Autodesk Inventor part; units mm, degrees
ref_plane "YZ Plane" through (0, 0, 0) normal (1, 0, 0) x (0, 1, 0)
ref_plane "XZ Plane" through (0, 0, 0) normal (0, 1, 0) x (-1, 0, 0)
ref_plane "XY Plane" through (0, 0, 0) normal (0, 0, 1) x (1, 0, 0)
ref_plane "Work Plane1" through (228.6, 0, -127) normal (0, 0, -1) x (-1, 0, 0)
sketch "Sketch5" plane through (228.6, 0, -127) normal (0, 0, -1) x (-1, 0, 0)
  line L0 (0, 0) -> (228.6, 0)
  line L1 (228.6, 0) -> (228.6, 194.818)
  line L2 (228.6, 194.818) -> (0, 194.818)
  line L3 (0, 194.818) -> (0, 0)
  circle A0 centre (549.0601, -0.0332) radius 2.1647 construction
  circle A1 centre (192.2498, 69.0594) radius 2.1647 construction
  arc A2 (37.5756, 109.1194) -> (31.2075, 73.1741) centre (549.0601, -0.0332) ccw construction
  arc A3 (33.8495, 109.9145) -> (27.435, 73.7074) centre (549.0601, -0.0332) ccw
  arc A4 (41.3017, 108.3242) -> (34.98, 72.6408) centre (549.0601, -0.0332) ccw
  arc A5 (41.3017, 108.3242) -> (33.8495, 109.9145) centre (37.5756, 109.1194) ccw
  arc A6 (27.435, 73.7074) -> (34.98, 72.6408) centre (31.2075, 73.1741) ccw
  line L4 (549.0601, -0.0332) -> (37.5756, 109.1194) construction
  line L5 (549.0601, -0.0332) -> (31.2075, 73.1741) construction
  arc A7 (14.9709, 119.3205) -> (7.984, 69.4017) centre (192.2498, 69.0594) ccw construction
  arc A8 (11.3053, 120.3597) -> (4.174, 69.4087) centre (192.2498, 69.0594) ccw
  arc A9 (18.6364, 118.2812) -> (11.794, 69.3946) centre (192.2498, 69.0594) ccw
  arc A10 (18.6364, 118.2812) -> (11.3053, 120.3597) centre (14.9709, 119.3205) ccw
  arc A11 (4.174, 69.4087) -> (11.794, 69.3946) centre (7.984, 69.4017) ccw
  circle A12 centre (192.2498, 69.0594) radius 2.1647
  circle A13 centre (216.5947, 65.3523) radius 2.2284
  line L6 (0, 0) -> (25.4, 0) construction
  line L7 (25.4, 0) -> (25.4, 25.4) construction
  line L8 (25.4, 25.4) -> (0, 25.4) construction
  line L9 (0, 25.4) -> (0, 0) construction
  line L10 (228.6, 0) -> (203.2, 0) construction
  line L11 (203.2, 0) -> (203.2, 25.4) construction
  line L12 (203.2, 25.4) -> (228.6, 25.4) construction
  line L13 (228.6, 25.4) -> (228.6, 0) construction
  line L14 (25.4, 25.4) -> (0, 0) construction
  line L15 (0, 25.4) -> (25.4, 0) construction
  line L16 (203.2, 25.4) -> (228.6, 0) construction
  line L17 (228.6, 25.4) -> (203.2, 0) construction
  circle A14 centre (12.7, 12.7) radius 2.3813
  circle A15 centre (215.9, 12.7) radius 2.3812
  line L18 (228.6, 194.818) -> (222.25, 194.818) construction
  line L19 (222.25, 194.818) -> (222.25, 169.418) construction
  line L20 (222.25, 169.418) -> (228.6, 169.418) construction
  line L21 (228.6, 169.418) -> (228.6, 194.818) construction
  line L22 (222.25, 194.818) -> (196.85, 194.818) construction
  line L23 (222.25, 169.418) -> (222.25, 194.818) construction
  line L24 (196.85, 194.818) -> (107.95, 194.818) construction
  line L25 (107.95, 194.818) -> (133.35, 194.818) construction
  line L26 (222.25, 194.818) -> (209.55, 194.818) construction
  line L27 (209.55, 194.818) -> (209.55, 182.118) construction
  line L28 (209.55, 182.118) -> (222.25, 182.118) construction
  line L29 (222.25, 182.118) -> (222.25, 194.818) construction
  line L30 (209.55, 194.818) -> (146.05, 194.818) construction
  line L31 (146.05, 194.818) -> (158.75, 194.818) construction
  line L32 (158.75, 194.818) -> (158.75, 182.118) construction
  line L33 (158.75, 182.118) -> (146.05, 182.118) construction
  line L34 (146.05, 182.118) -> (146.05, 194.818) construction
  line L35 (222.25, 194.818) -> (209.55, 182.118) construction
  line L36 (209.55, 194.818) -> (222.25, 182.118) construction
  line L37 (158.75, 194.818) -> (146.05, 182.118) construction
  line L38 (158.75, 182.118) -> (146.05, 194.818) construction
  circle A16 centre (215.9, 188.468) radius 2.3812
  circle A17 centre (152.4, 188.468) radius 2.3812
  dimension "d16" = 228.6
  dimension "d17" = 194.818
  dimension "d38" = 4
  dimension "d39" = 7.62
  dimension "d40" = 7.62
  dimension "d43" = 25.4
  dimension "d44" = 25.4
  dimension "d45" = 25.4
  dimension "d46" = 25.4
  dimension "d47" = 4.7625
  dimension "d48" = 4.7625
  dimension "d61" = 6.35
  dimension "d70" = 12.7
  dimension "d71" = 12.7
  dimension "d72" = 63.5
  dimension "d73" = 12.7
  dimension "d74" = 12.7
  dimension "d75" = 4.7625
  dimension "d76" = 4.7625
extrude "Extrusion5" add sketch "Sketch5" along normal blind 3.175
ref_plane "Work Plane2" through (0, 0.0003, -127) normal (-1, 0, 0) x (0, 0, 1)
sketch "Sketch6" plane through (0, 0.0003, -127) normal (-1, 0, 0) x (0, 0, 1)
  line L0 (-3.175, -0.0003) -> (-3.175, 194.8177)
  line L1 (-3.175, 194.8177) -> (127, 194.8177)
  line L2 (127, 194.8177) -> (127, -0.0003)
  line L3 (127, -0.0003) -> (-3.175, -0.0003)
  line L4 (-3.175, -0.0003) -> (-3.175, 194.8177)
  line L5 (0, -0.0003) -> (0, 194.8177) construction
  line L6 (0, -0.0003) -> (25.4, -0.0003) construction
  line L7 (25.4, -0.0003) -> (25.4, 25.3997) construction
  line L8 (25.4, 25.3997) -> (0, 25.3997) construction
  line L9 (0, 25.3997) -> (0, -0.0003) construction
  line L10 (127, -0.0003) -> (101.6, -0.0003) construction
  line L11 (101.6, -0.0003) -> (101.6, 25.3997) construction
  line L12 (101.6, 25.3997) -> (127, 25.3997) construction
  line L13 (127, 25.3997) -> (127, -0.0003) construction
  line L14 (0, -0.0003) -> (25.4, 25.3997) construction
  line L15 (0, 25.3997) -> (25.4, -0.0003) construction
  line L16 (101.6, -0.0003) -> (127, 25.3997) construction
  line L17 (101.6, 25.3997) -> (127, -0.0003) construction
  circle A0 centre (12.7, 12.6997) radius 2.3813
  circle A1 centre (114.3, 12.6997) radius 2.3813
  line L18 (0, 194.8177) -> (3.175, 194.8177) construction
  line L19 (3.175, 194.8177) -> (3.175, 169.4177) construction
  line L20 (3.175, 169.4177) -> (0, 169.4177) construction
  line L21 (0, 169.4177) -> (0, 194.8177) construction
  line L22 (3.175, 194.8177) -> (15.875, 194.8177) construction
  line L23 (15.875, 194.8177) -> (15.875, 182.1177) construction
  line L24 (15.875, 182.1177) -> (3.175, 182.1177) construction
  line L25 (3.175, 182.1177) -> (3.175, 194.8177) construction
  line L26 (15.875, 194.8177) -> (104.775, 194.8177) construction
  line L27 (104.775, 194.8177) -> (92.075, 194.8177) construction
  line L28 (92.075, 194.8177) -> (92.075, 182.1177) construction
  line L29 (92.075, 182.1177) -> (104.775, 182.1177) construction
  line L30 (104.775, 182.1177) -> (104.775, 194.8177) construction
  line L31 (3.175, 194.8177) -> (15.875, 182.1177) construction
  line L32 (3.175, 182.1177) -> (15.875, 194.8177) construction
  line L33 (92.075, 194.8177) -> (104.775, 182.1177) construction
  line L34 (104.775, 194.8177) -> (92.075, 182.1177) construction
  circle A2 centre (98.425, 188.4677) radius 2.3812
  circle A3 centre (9.525, 188.4677) radius 2.3813
  point P0 (-3.175, -0.0003)
  dimension "d49" = 25.4
  dimension "d50" = 25.4
  dimension "d51" = 25.4
  dimension "d52" = 25.4
  dimension "d53" = 4.7625
  dimension "d54" = 4.7625
  dimension "d77" = 3.175
  dimension "d78" = 25.4
  dimension "d79" = 12.7
  dimension "d80" = 12.7
  dimension "d81" = 88.9
  dimension "d82" = 12.7
  dimension "d83" = 12.7
  dimension "d84" = 4.7625
  dimension "d85" = 4.7625
extrude "Extrusion6" add sketch "Sketch6" along normal blind 3.175
ref_plane "Work Plane4" through (0, 0.0003, 0) normal (0, 0, 1) x (1, 0, 0)
sketch "Sketch7" plane through (0, 0.0003, 0) normal (0, 0, 1) x (1, 0, 0)
  line L0 (228.6, -0.0003) -> (228.6, 0)
  line L1 (228.6, -0.0003) -> (127, -0.0003)
  line L2 (127, -0.0003) -> (127, 194.8177)
  line L3 (127, 194.8177) -> (228.6, 194.8177)
  line L4 (228.6, 194.8177) -> (228.6, -0.0003)
  line L5 (228.6, -0.0003) -> (-3.175, -0.0003)
  line L6 (228.6, -0.0003) -> (127, -0.0003)
  line L7 (127, -0.0003) -> (127, 133.3497)
  line L8 (127, 133.3497) -> (228.6, 133.3497)
  line L9 (228.6, 133.3497) -> (228.6, -0.0003)
  arc A0 (217.2947, 120.3594) -> (209.9636, 118.281) centre (213.6291, 119.3202) ccw
  arc A1 (216.806, 69.3943) -> (209.9636, 118.281) centre (36.3502, 69.0591) ccw
  arc A2 (224.426, 69.4085) -> (217.2947, 120.3594) centre (36.3502, 69.0591) ccw
  arc A3 (216.806, 69.3943) -> (224.426, 69.4085) centre (220.616, 69.4014) ccw
  arc A4 (194.7505, 109.9143) -> (187.2983, 108.324) centre (191.0244, 109.1191) ccw
  arc A5 (193.62, 72.6406) -> (187.2983, 108.324) centre (-320.4601, -0.0334) ccw
  arc A6 (201.165, 73.7072) -> (194.7505, 109.9143) centre (-320.4601, -0.0334) ccw
  arc A7 (193.62, 72.6406) -> (201.165, 73.7072) centre (197.3925, 73.1739) ccw
  line L10 (127, -0.0003) -> (152.4, -0.0003) construction
  line L11 (152.4, -0.0003) -> (152.4, 25.3997) construction
  line L12 (152.4, 25.3997) -> (127, 25.3997) construction
  line L13 (127, 25.3997) -> (127, -0.0003) construction
  line L14 (228.6, 194.8177) -> (228.6, -0.0003) construction
  line L15 (228.6, -0.0003) -> (203.2, -0.0003) construction
  line L16 (203.2, -0.0003) -> (203.2, 25.3997) construction
  line L17 (203.2, 25.3997) -> (228.6, 25.3997) construction
  line L18 (228.6, 25.3997) -> (228.6, -0.0003) construction
  line L19 (127, 25.3997) -> (152.4, -0.0003) construction
  line L20 (152.4, 25.3997) -> (127, -0.0003) construction
  line L21 (228.6, -0.0003) -> (-3.175, -0.0003) construction
  line L22 (203.2, 25.3997) -> (228.6, -0.0003) construction
  line L23 (228.6, -0.0003) -> (228.6, 25.3997) construction
  line L24 (228.6, 25.3997) -> (203.2, -0.0003) construction
  circle A8 centre (139.7, 12.6997) radius 2.3813
  circle A9 centre (215.9, 12.6997) radius 2.3813
  line L25 (0, -0.0003) -> (0, 194.8177)
  line L26 (0, 121.2789) -> (127, 121.2789)
  line L27 (127, 121.2789) -> (127, 104.7109)
  line L28 (0, 104.7109) -> (0, 121.2789)
  line L29 (127, 133.3497) -> (100.9092, 133.3497)
  line L30 (100.9092, 133.3497) -> (100.9092, 121.2789)
  line L31 (100.9092, 121.2789) -> (127, 121.2789)
  line L32 (127, 121.2789) -> (127, 133.3497)
  line L33 (0, 121.2789) -> (127, 121.2789)
  line L34 (127, 121.2789) -> (127, 81.6877)
  line L35 (127, 81.6877) -> (0, 81.6877)
  line L36 (0, 81.6877) -> (0, 121.2789)
  line L37 (0, 121.2789) -> (-3.175, 121.2789)
  line L38 (-3.175, 121.2789) -> (-3.175, 81.6877)
  line L39 (-3.175, 81.6877) -> (0, 81.6877)
  line L40 (0, 81.6877) -> (0, 121.2789)
  point P0 (127, 133.3497)
  dimension "d22" = 101.6
  dimension "d23" = 194.818
  dimension "d26" = 101.6
  dimension "d27" = 133.35
  dimension "d55" = 25.4
  dimension "d56" = 25.4
  dimension "d57" = 25.4
  dimension "d58" = 25.4
  dimension "d59" = 4.7625
  dimension "d60" = 4.7625
extrude "Extrusion7" add sketch "Sketch7" along normal blind 3.175 contours L1 L2 L8 L4 | L35 L25 L26 L2 | L2 L26 L30 L29 | L39 L38 L37 L25
ref_plane "Work Plane3" through (0, 0.0003, 0) normal (0, 0, 1) x (1, 0, 0)
sketch "Sketch8" plane through (0, 0.0003, 0) normal (0, 0, 1) x (1, 0, 0)
  line L0 (18.6832, 91.7066) -> (0, 110.3898)
  line L1 (0, 0) -> (0, 194.8177)
  line L2 (18.6832, 91.7066) -> (45.1053, 91.7066) construction
  line L3 (0, 110.3898) -> (0, 113.5648) construction
  line L4 (0, 113.5648) -> (21.8582, 91.7066)
  line L5 (0, 113.5648) -> (0, 110.3898) construction
  line L6 (18.6832, 91.7066) -> (21.8582, 91.7066) construction
  line L7 (18.6832, 91.7066) -> (21.8582, 91.7066)
  line L8 (0, 113.5648) -> (0, 110.3898)
  line L9 (18.6832, 91.7066) -> (16.4382, 93.9517)
  line L10 (18.6832, 91.7066) -> (21.8582, 91.7066) construction
  line L11 (18.6832, 91.7066) -> (0, 91.7066)
  line L12 (18.6832, 91.7066) -> (37.3664, 91.7066) construction
  line L13 (0, 91.7066) -> (0, 94.8816)
  line L14 (0, 94.8816) -> (15.5082, 94.8816)
  point P0 (0, -0.0003)
  dimension "d28" = 135
  dimension "d29" = 3.175
  dimension "d30" = 45
  dimension "d31" = 3.175
  dimension "d32" = 135
  dimension "d33" = 180
  dimension "d34" = 3.175
  dimension "d35" = 90
extrude "Extrusion8" [suppressed]
sketch "Sketch10" plane through (228.6, 0, -127) normal (0, 0, 1) x (1, 0, 0)
  line L0 (0, 0) -> (-25.4, 0) construction
  line L1 (0, 0) -> (25.4, 0) construction
  line L2 (-25.4, 0) -> (-28.575, 0)
  line L3 (-28.575, 0) -> (-28.575, 38.1)
  line L4 (-28.575, 38.1) -> (-25.4, 38.1)
  line L5 (-25.4, 38.1) -> (-25.4, 0)
  point P0 (-228.6, 0)
  dimension "d86" = 25.4
  dimension "d87" = 180
  dimension "d88" = 3.175
  dimension "d89" = 38.1
extrude "Extrusion9" add sketch "Sketch10" along normal blind 127
properties part number "ShootingMech_Housing6"
Build history of the part. All positions in model axes, mm. A direction names the side the tool comes from. Coordinates: 2 decimals unless noted, no trailing zeros. Write each loop counter-clockwise with the first axis right and the second up, starting at its lowest first coordinate (ties: lowest second). Pieces come first, ordered by that corner, then holes.
(1) 3-axis set-ups, long thin cutter, end or side, ignore diameter. For faces 4 (the flat face through (200.025, 19, -64)), 5 (the flat face through (-3.175, 99, -64)), 6 (the cylindrical face through (215.016, 94.416, 1.565)), 7 (the flat face through (203.2, 19, -64)): which of +Z, -Z, +X, -X, +Y, -Y reach the whole face in a straight line?
(2) Pin check, flat tips, straight feed: pin 1 Ø1.6 at (x, z) = (86.5, 1) entering from -Y; pin 2 Ø4 at (x, y) = (139.7, 12.7) entering from +Z; pin 3 Ø2.5 at (x, z) = (62, 1.5) entering from +Y. Stop position of each tip, or through.
(3) Mould opens along Y. For faces 1 (the cylindrical face through (190.815, 90.288, -128.565)), 2 (the flat face through (138, 82, 0)), 3 (the flat face through (112.2, 194.818, -127.5)) say: pulls with the +Y half, pulls with the -Y half, needs draft (parallel to the pull), parting line crosses it, or undercut.
(4) Cut at D-D on x = 190.5. List the corners of the cut face in (y, z) (3 decimals), and give its area (3 significant figures).
(5) Cut at A-A on x = 45. List the corners of the cut face in (y, z) (3 decimals), and give its area (3 significant figures).
(6) Drill centre lines: line 1 (Y direction, x = -1.65, z = -12.7); line 2 (Y direction, x = 76, z = -129); line 3 (X direction, y = 22.5, z = -2.5) (3 decimals). Where is each one in solid material? Low to high.
(7) Cut at B-B on z = -108. List the corners of the cut face in (x, y) (3 decimals), and give its area (3 significant figures).
(8) Cut at C-C on y = 144. List the corners of the cut face in (x, z) (3 decimals), and give its area (3 significant figures).
Working result:
1. face 4: +Y, -Y
1. face 5: +Z, -Z, -X, +Y, -Y
1. face 6: +Z, -Z
1. face 7: +X, +Y, -Y
2. pin 1: stops at y = 81.69
2. pin 2: stops at z = -127
2. pin 3: stops at y = 121.28
3. face 1: undercut
3. face 2: needs draft
3. face 3: pulls with the +Y half
4. outline: (0, -130.175) - (92.052, -130.175) - (92.052, -127) - (0, -127) - close; (0, 0) - (92.052, 0) - (92.052, 3.175) - (0, 3.175) - close; (112.893, -130.175) - (194.818, -130.175) - (194.818, -127) - (112.893, -127) - close; (112.893, 0) - (133.35, 0) - (133.35, 3.175) - (112.893, 3.175) - close
4. area: 910 mm2
5. outline: (0, -130.175) - (194.818, -130.175) - (194.818, -127) - (0, -127) - close; (81.688, 0) - (121.279, 0) - (121.279, 3.175) - (81.688, 3.175) - close
5. area: 744 mm2
6. line 1: y = 0 to 10.32, 15.08 to 194.82
6. line 2: y = 0 to 186.1, 190.84 to 194.82
6. line 3: x = -3.175 to 0, 200.025 to 203.2
7. outline: (-3.175, 0) - (0, 0) - (0, 194.818) - (-3.175, 194.818) - close; (200.025, 0) - (203.2, 0) - (203.2, 38.1) - (200.025, 38.1) - close
7. area: 740 mm2
8. outline: (-3.175, -130.175) - (228.6, -130.175) - (228.6, -127) - (0, -127) - (0, 0) - (-3.175, 0) - close
8. area: 1,140 mm2
